Input: part model. Units: mm. Frame: model coordinates. Face numbers are marked on the shaded views. A direction names the side the tool comes from. Give positions to 0.01 mm unless a question says otherwise; leave off trailing zeros. Write each loop counter-clockwise with the first axis right and the second up, starting at its lowest first coordinate (ties: lowest second). Pieces come first, ordered by that corner, then holes. Notation, with made-up numbers: (27, -5.75) -> (61, -5.75) arc R28 cw to (61, 21.25) -> close; hole circle Ø7 at (-37, 47.5). An arc over 180 degrees is marked (long way). Return JSON: item names as keys, results as strings. Group by question number.
Item 1: Set-up query: the marked faces 1, 2, 3, 4 and 5. Return all of +Z, -Z, +X, -X, +Y, -Y with unobstructed straight access to the full face (end or side cutting, diameter ignored); none if empty.
Item 2: Section A-A, the plane y = -3.25. Return loops of the section in (x, z) (3 decimals).
Item 3: Section D-D, the plane z = -1.35. Return loops of the section in (x, y) (3 decimals), then the cut area to 3 significant figures.
Item 4: Pin query (flat end, axial travel): P1, Ø2.5, axis at y = 0, z = -1.5, coming from the +X side; P2, Ø0.6, axis at x = 7.5, z = -1, coming from the -Y side (3 decimals); P3, Ø2.5, axis at y = -4, z = -2, coming from the +X side; P4, Ø2.5, axis at y = -6, z = -1, coming from the -X side. Return the tip coordinate at first contact, or that it passes through.
Item 5: Section B-B, the plane z = 1.85. Return loops of the section in (x, y) (3 decimals).
Item 6: Mould query, pull axis X, two halves, no side actions, for the marked faces 6, 7 and 8. Classes: released by +X, released by -X, zero draft, split by the parting line, or undercut.
Item 7: Line query: line 1 (X direction, y = -3.25, z = 1.25) (3 decimals); line 2 (Y direction, x = 9, z = 1.5) (3 decimals); line 3 (X direction, y = -5.25, z = -0.7). Output: solid intervals per line, ascending. Write a range as [from, to].
Item 8: Section C-C, the plane x = -9. Return loops of the section in (y, z) (3 decimals), then the cut area to 3 significant figures.
from build123d import *

# Parameters (mm, degrees)
F0_W      = 23
F0_H      = 9.25
F1_DEPTH  = 3
F3_DEPTH  = 3.6
F4_W      = 11
F4_H      = 3.5
F5_DEPTH  = 6.601
F7_DEPTH  = 0.75
F8_DEPTH  = 3.501
F9_DEPTH  = 3.5
F11_DEPTH = 3
F12_R     = 1.625
F13_DEPTH = 3.001


with BuildPart() as f1:
    # F0 (on Top) → F1 (new body)
    with BuildSketch(Plane.XY):
        Rectangle(F0_W, F0_H)
    extrude(amount=F1_DEPTH)

    # F2 (on face) → F3 (join)
    with BuildSketch(Plane(origin=(0, 0, 0), x_dir=(1, 0, 0), z_dir=(0, 0, -1))):
        Polygon((7, 4.625), (-7, 4.625), (-7, 1.125), (-8.25, 1.125), (-8.25, -1.125), (-5.5, -1.125), (-5.5, -4.625), (5.5, -4.625), (5.5, -1.125), (8.25, -1.125), (8.25, 1.125), (7, 1.125), align=None)
    extrude(amount=F3_DEPTH)

    # F4 (on face) → F5 (cut, through all)
    with BuildSketch(Plane(origin=(0, 0, -3.6), x_dir=(1, 0, 0), z_dir=(0, 0, -1))):
        with Locations((0, -2.875)):
            Rectangle(F4_W, F4_H)
    extrude(amount=-F5_DEPTH, mode=Mode.SUBTRACT)

    # F6 (on face) → F7 (cut)
    with BuildSketch(Plane(origin=(0, 0, -3.6), x_dir=(1, 0, 0), z_dir=(0, 0, -1))):
        Polygon((-8.25, -1.125), (8.25, -1.125), (8.25, 1.125), (7, 1.125), (-7, 1.125), (-8.25, 1.125), align=None)
    extrude(amount=-F7_DEPTH, mode=Mode.SUBTRACT)

    # F8 (cut, through all): a face of the model
    f8_faces = [f1.faces().sort_by_distance(p)[0] for p in [
        (0, -1.125, -3.225),
    ]]
    extrude(f8_faces, amount=-F8_DEPTH, mode=Mode.SUBTRACT)

    # F9 (add): a face of the model
    f9_faces = [f1.faces().sort_by_distance(p)[0] for p in [
        (0, -4.625, 0.4283057851),
    ]]
    extrude(f9_faces, amount=F9_DEPTH)

    # F10 (on face) → F11 (join)
    with BuildSketch(Plane.XZ.offset(8.125)):
        Polygon((11.5, 3), (-11.5, 3), (-11.5, 0), (-7, 0), (7, 0), (11.5, 0), align=None)
    extrude(amount=F11_DEPTH)

    # F12 (on face) → F13 (cut, through all)
    with BuildSketch(Plane(origin=(0, 0, 0), x_dir=(1, 0, 0), z_dir=(0, 0, -1))):
        with Locations((-9, 3.25)):
            Circle(F12_R)
        with Locations((9, 3.25)):
            Circle(F12_R)
    extrude(amount=-F13_DEPTH, mode=Mode.SUBTRACT)


solid = f1.part
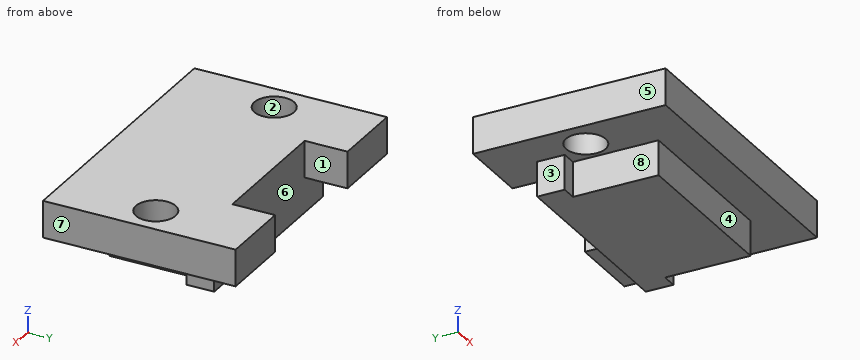
Answer below:
{
 "1": {"face 1": "+Z, -Z, +Y", "face 2": "+Z, -Z", "face 3": "-Z, -X, +Y, -Y", "face 4": "-Z, +X, -X, -Y", "face 5": "+Z, -Z, -X, +Y, -Y"},
 "2": {"outline": "(-11.5, 0) -> (-10.625, 0) -> (-10.625, 3) -> (-11.5, 3) -> close; (-7.375, 0) -> (-7, 0) -> (-7, -2.85) -> (7, -2.85) -> (7, 0) -> (7.375, 0) -> (7.375, 3) -> (-7.375, 3) -> close; (10.625, 0) -> (11.5, 0) -> (11.5, 3) -> (10.625, 3) -> close"},
 "3": {"outline": "(-8.25, -1.125) -> (-7, -1.125) -> (-7, -8.125) -> (7, -8.125) -> (7, -1.125) -> (8.25, -1.125) -> (8.25, 1.125) -> (-8.25, 1.125) -> close", "area": "135 mm2"},
 "4": {"P1": "stops at x = 8.25", "P2": "stops at y = -1.125", "P3": "stops at x = 7", "P4": "stops at x = -11.5"},
 "5": {"outline": "(-11.5, -11.125) -> (11.5, -11.125) -> (11.5, 4.625) -> (5.5, 4.625) -> (5.5, 1.125) -> (-5.5, 1.125) -> (-5.5, 4.625) -> (-11.5, 4.625) -> close; hole circle Ø3.25 at (-9, -3.25); hole circle Ø3.25 at (9, -3.25)"},
 "6": {"face 6": "undercut", "face 7": "released by +X", "face 8": "released by -X"},
 "7": {"line 1": "x = [-11.5, -10.625], [-7.375, 7.375], [10.625, 11.5]", "line 2": "y = [-11.125, -4.875], [-1.625, 4.625]", "line 3": "x = [-7, 7]"},
 "8": {"outline": "(-11.125, 0) -> (-4.875, 0) -> (-4.875, 3) -> (-11.125, 3) -> close; (-1.625, 0) -> (4.625, 0) -> (4.625, 3) -> (-1.625, 3) -> close", "area": "37.5 mm2"}
}
